Read the model definition and answer for the solid it produces. Units are mm, in the model's axes. Face numbers are marked on the shaded views. A direction names the side the tool comes from. Coordinates: 2 decimals unless noted, no trailing zeros. Loops run counter-clockwise (first coordinate to the right, second up) from the corner with the lowest first, then second, coordinate; pieces in that order, holes last.
Q1. Section B-B (x = 5.8) is taken. Give the vertices of the cut face in (y, z), then the cut area to 3 significant figures.
Q2. Which of the six approach directions +Z, -Z, +X, -X, +Y, -Y give full straight-line access (tool end or side, diameter ignored) to the marked faces 1, 2 and 3?
Q3. Straight lines are drawn through the part: line 1 (X direction, y = 1.45, z = 9); line 2 (Y direction, x = 6, z = 2); line 3 (Y direction, x = 23, z = 9.25). For each, find the intervals that lie inside material, in ascending order.
Q4. Section D-D (z = 1.75) is taken. Give the vertices of the cut face in (x, y), then the cut area to 3 significant figures.
Q5. Flat-ended cylindrical pins translate along their axes: P1, Ø3, axis at x = 5.8, z = 9, coming from the -Y side; P2, Ø5, axis at x = 6, y = 10, coming from the +Z side; P3, Ø4, axis at x = 36.2, z = 9, coming from the +Y side. Find the tip coordinate at first contact, or state that the pin passes through.
Q6. Section C-C (y = 10.5) is taken. Give the vertices of the cut face in (x, z).
Q7. Section A-A (z = 9.5) is taken. Give the vertices of the cut face in (x, y), then the cut area to 3 significant figures.
from build123d import *

# Parameters (mm, degrees)
SKETCH1_W           = 42
SKETCH1_H           = 3
BOSS_EXTRUDE1_DEPTH = 15
SKETCH2_W           = 42
SKETCH2_H           = 3
BOSS_EXTRUDE2_DEPTH = 17
CUT_EXTRUDE1_REACH  = 49.728
SKETCH6_R           = 1.6
CUT_EXTRUDE2_REACH  = 50.877
SKETCH7_R           = 1.6
BOSS_EXTRUDE3_DEPTH = 1.5
FILLET1_R           = 10


with BuildPart() as part:
    # Sketch1 → Boss-Extrude1 (new body)
    with BuildSketch(Plane.XY):
        with Locations((21, 1.5)):
            Rectangle(SKETCH1_W, SKETCH1_H)
    extrude(amount=BOSS_EXTRUDE1_DEPTH)

    # Sketch2 → Boss-Extrude2 (add)
    with BuildSketch(Plane(origin=(0, 3, 0), x_dir=(1, 0, 0), z_dir=(0, 1, 0))):
        with Locations((21, -1.5)):
            Rectangle(SKETCH2_W, SKETCH2_H)
    extrude(amount=BOSS_EXTRUDE2_DEPTH)

    # Sketch6 → Cut-Extrude1 (cut, up to next)
    with BuildSketch(Plane(origin=(0, 3, 0), x_dir=(1, 0, 0), z_dir=(0, 1, 0)), mode=Mode.PRIVATE) as cut_extrude1_sk1:
        with Locations(Location((5.8, -9, 0), (0, 0, 270))):
            Circle(SKETCH6_R)
    cut_extrude1_tool1 = extrude(cut_extrude1_sk1.sketch, amount=-CUT_EXTRUDE1_REACH, mode=Mode.PRIVATE) & part.part
    # Sketch6 → Cut-Extrude1 (cut, up to next)
    with BuildSketch(Plane(origin=(0, 3, 0), x_dir=(1, 0, 0), z_dir=(0, 1, 0)), mode=Mode.PRIVATE) as cut_extrude1_sk2:
        with Locations(Location((36.2, -9, 0), (0, 0, 270))):
            Circle(SKETCH6_R)
    cut_extrude1_tool2 = extrude(cut_extrude1_sk2.sketch, amount=-CUT_EXTRUDE1_REACH, mode=Mode.PRIVATE) & part.part
    add(cut_extrude1_tool1.solids().sort_by_distance((5.8, 3, 9))[0], mode=Mode.SUBTRACT)
    add(cut_extrude1_tool2.solids().sort_by_distance((36.2, 3, 9))[0], mode=Mode.SUBTRACT)

    # Sketch7 → Cut-Extrude2 (cut, up to next)
    with BuildSketch(Plane(origin=(0, 0, 0), x_dir=(-1, 0, 0), z_dir=(0, 0, -1)), mode=Mode.PRIVATE) as cut_extrude2_sk1:
        with Locations((-36, 10)):
            Circle(SKETCH7_R)
    cut_extrude2_tool1 = extrude(cut_extrude2_sk1.sketch, amount=-CUT_EXTRUDE2_REACH, mode=Mode.PRIVATE) & part.part
    # Sketch7 → Cut-Extrude2 (cut, up to next)
    with BuildSketch(Plane(origin=(0, 0, 0), x_dir=(-1, 0, 0), z_dir=(0, 0, -1)), mode=Mode.PRIVATE) as cut_extrude2_sk2:
        with Locations((-6, 10)):
            Circle(SKETCH7_R)
    cut_extrude2_tool2 = extrude(cut_extrude2_sk2.sketch, amount=-CUT_EXTRUDE2_REACH, mode=Mode.PRIVATE) & part.part
    add(cut_extrude2_tool1.solids().sort_by_distance((36, 10, 0))[0], mode=Mode.SUBTRACT)
    add(cut_extrude2_tool2.solids().sort_by_distance((6, 10, 0))[0], mode=Mode.SUBTRACT)

    # Sketch9 → Boss-Extrude3 (add, symmetric)
    with BuildSketch(Plane.ZY.offset(-21)):
        Polygon((3, 10.323968285), (10.323968285, 3), (3, 3), align=None)
    extrude(amount=BOSS_EXTRUDE3_DEPTH, both=True)

    # Fillet1
    fillet1_edges = [part.edges().sort_by_distance(p)[0] for p in [
        (21, 10.323968285, 3),
        (21, 3, 10.323968285),
    ]]
    fillet(fillet1_edges, radius=FILLET1_R)


solid = part.part
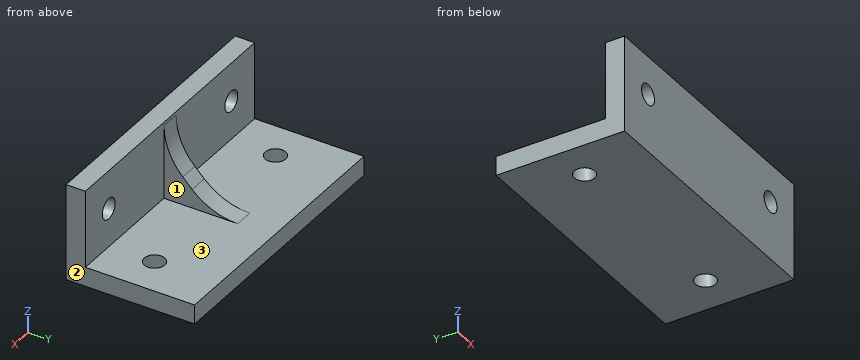
Numbers:
1. outline: (0, 0) - (8.41, 0) - (8.41, 3) - (3, 3) - (3, 7.4) - (0, 7.4) - close; (0, 10.6) - (3, 10.6) - (3, 15) - (0, 15) - close; (11.59, 0) - (20, 0) - (20, 3) - (11.59, 3) - close
1. area: 76.9 mm2
2. face 1: +Z, +X, +Y
2. face 2: +Z, -Z, +X, +Y, -Y
2. face 3: +Z, +Y
3. line 1: x = 0 to 4.2, 7.4 to 34.6, 37.8 to 42
3. line 2: y = 0 to 8.4, 11.6 to 20
3. line 3: y = 0 to 3
4. outline: (0, 0) - (42, 0) - (42, 20) - (0, 20) - close; hole circle Ø3.2 at (6, 10); hole circle Ø3.2 at (36, 10)
4. area: 824 mm2
5. P1: passes through
5. P2: stops at z = 3
5. P3: stops at y = 3
6. outline: (0, 0) - (4.48, 0) - (4.48, 3) - (0, 3) - close; (7.52, 0) - (34.48, 0) - (34.48, 3) - (22.5, 3) - (22.5, 3.82) - (19.5, 3.82) - (19.5, 3) - (7.52, 3) - close; (37.52, 0) - (42, 0) - (42, 3) - (37.52, 3) - close
7. outline: (0, 0) - (4.28, 0) - (4.28, 3) - (0, 3) - close; (7.32, 0) - (34.68, 0) - (34.68, 3) - (22.5, 3) - (22.5, 4.32) - (19.5, 4.32) - (19.5, 3) - (7.32, 3) - close; (37.72, 0) - (42, 0) - (42, 3) - (37.72, 3) - close
7. area: 112 mm2
